Here's the drawing with two shaded views (mm, measured from the low corner). I have some questions. Coordinates: 2 decimals unless noted, no trailing zeros. Loops run counter-clockwise (first coordinate to the right, second up) from the corner with the lowest first, then second, coordinate; pieces in that order, holes last. Notation, with made-up numbers: (68.25, 61) -> (75.25, 61) arc R20 ccw to (75.25, 72) -> close; hole circle Ø5 at (-12, -24). An arc over 180 degrees is marked (long way). Answer as a JSON object with one key per item and string values. Group by question number.
Q1. I'm going to push flat-ended pins straight in: pin 1 (1.5 mm diameter, centred on x = 15.5, y = 30, fed in from -Z); pin 2 (8.5 mm diameter, centred on x = 18.77, z = 10.16, fed in from -Y); pin 3 (10 mm diameter, centred on y = 47.5, z = 11.5, fed in from -X); pin 4 (3 mm diameter, centred on y = 24, z = 10, fed in from +X). Where does each tip first touch, or does it pass through?
Q2. I want a section at B-B on y = 16. Write out the boundary of the cut face in (x, z) (3 decimals), then the cut area to 3 significant figures.
Q3. I want a section at C-C on x = 79. Write out the boundary of the cut face in (y, z), then the cut area to 3 significant figures.
Q4. I want a section at A-A on z = 10.16. Write out the boundary of the cut face in (x, y), then the cut area to 3 significant figures.
Q5. I need wall thicknesses on line 1 (X direction, y = 16, z = 10.16); line 2 (X direction, y = 31, z = 9); line 3 (Y direction, x = 74, z = 18.25). Which ranges of each line are inside material? Lowest first, please.
Q6. Thinking about a two-plate mould opening in X: for the marked faces 1 and 2, which applies, released by +X, released by -X, zero draft, split by the parting line, or undercut?
Q7. I want a section at D-D on z = 1.75. Write out the boundary of the cut face in (x, y).
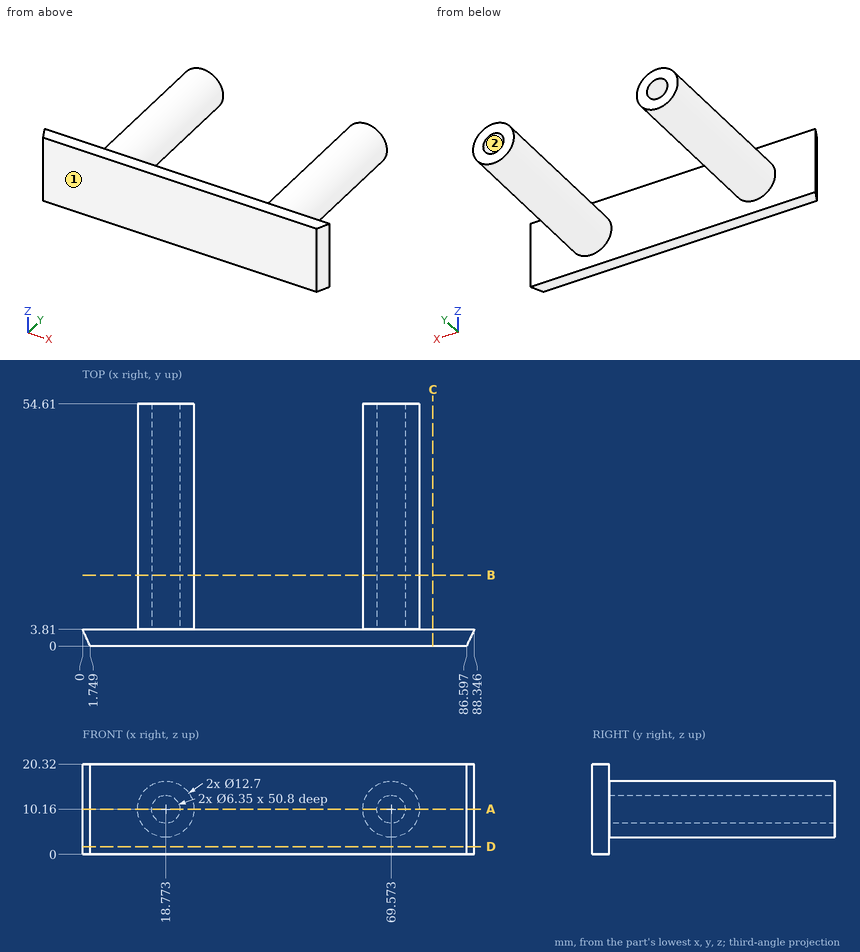
Result set:
{
 "1": {"pin 1": "stops at z = 4.33", "pin 2": "stops at y = 0", "pin 3": "stops at x = 12.42", "pin 4": "stops at x = 75.92"},
 "2": {"outline": "circle Ø12.7 at (18.773, 10.16); circle Ø12.7 at (69.573, 10.16); hole circle Ø6.35 at (18.773, 10.16); hole circle Ø6.35 at (69.573, 10.16)", "area": "190 mm²"},
 "3": {"outline": "(0, 0) -> (3.81, 0) -> (3.81, 20.32) -> (0, 20.32) -> close", "area": "77.4 mm²"},
 "4": {"outline": "(0, 3.81) -> (1.75, 0) -> (86.6, 0) -> (88.35, 3.81) -> (75.92, 3.81) -> (75.92, 54.61) -> (72.75, 54.61) -> (72.75, 3.81) -> (66.4, 3.81) -> (66.4, 54.61) -> (63.22, 54.61) -> (63.22, 3.81) -> (25.12, 3.81) -> (25.12, 54.61) -> (21.95, 54.61) -> (21.95, 3.81) -> (15.6, 3.81) -> (15.6, 54.61) -> (12.42, 54.61) -> (12.42, 3.81) -> close", "area": "975 mm²"},
 "5": {"line 1": "x = 12.42 to 15.6, 21.95 to 25.12, 63.22 to 66.4, 72.75 to 75.92", "line 2": "x = 12.53 to 15.82, 21.73 to 25.02, 63.33 to 66.62, 72.53 to 75.82", "line 3": "y = 0 to 3.81"},
 "6": {"face 1": "zero draft", "face 2": "undercut"},
 "7": {"outline": "(0, 3.81) -> (1.75, 0) -> (86.6, 0) -> (88.35, 3.81) -> close"}
}
